For this review, take the finished solid that the model builds, in its own axes (mm). Face numbers are marked on the shaded views. A direction names the side the tool comes from. Coordinates: 2 decimals unless noted, no trailing zeros. Loops run counter-clockwise (first coordinate to the right, second up) from the corner with the lowest first, then second, coordinate; pieces in that order, holes last. Notation, with made-up numbers: M -24,74.5 L -4,74.5 A20 ccw -4,91.5 Z; hole C 24.25,25.25 d8. An arc over 180 degrees is marked long. Answer as a JSON object with one key per item and string values. Group by question number.
Item 1: Wall thickness on L1, parallel to Z at x = 8, y = -19.5; L2, parallel to Y at x = 38, z = 17.5; L3, parallel to X at y = -11, z = 24: over which ranges is each line inside the solid? List them lowest first. Write a range as from..to.
Item 2: Tool access review of the marked faces 4 and 5: name each direction out of +Z, -Z, +X, -X, +Y, -Y from which nothing blocks a thin tool from reaching the whole face with its end or side.
Item 3: Add section A-A (y = -20). State the section outline as (x, z) points.
Item 4: Add section B-B (x = -27.5). State the section outline as (y, z) points, then the cut area to 3 significant figures.
Item 5: Add section C-C (x = 3.5). State the section outline as (y, z) points.
Item 6: Mouldability with a two-part tool opening along X and no side actions: class the marked faces 1, 2 and 3 as +X half, -X half, draft (parallel to the pull), parting line (faces both ways), or undercut.
Item 7: Add section D-D (y = 8.5). State the section outline as (x, z) points, then the cut area to 3 significant figures.
Item 8: Insertion check: pin 1 (3 mm diameter, centred on y = -12.5, z = 30.5, fed in from -X); pin 2 (4 mm diameter, centred on y = -21.5, z = 22.5, fed in from +X); pin 3 (10 mm diameter, centred on x = -1.5, y = -19.5, fed in from -Z). Each pin has a flat end and moves straight along its axis. Give the tip position at first contact, or say it passes through.
from build123d import *

# Parameters (mm, degrees)
F1_DEPTH  = 12.7
F2_DEPTH  = 12.7
F3_R      = 3.8439536327
F4_DEPTH  = 25.401
F5_W      = 29.3294070289
F5_H      = 13.9285232872
F6_DEPTH  = 12.7
F8_DEPTH  = 18.6216022351
F9_R      = 3.0824278946
F10_DEPTH = 59.0766736131


with BuildPart() as f1:
    # F0 (on Front) → F1 (new body, symmetric)
    with BuildSketch(Plane.XZ):
        with BuildLine():
            Line((35.185629891, 37.1372154056), (-28.314370109, 37.1372154056))
            ThreePointArc((-28.314370109, 37.1372154056), (-19.6745097456, 33.5584680661), (-16.0957624062, 24.9186077028))
            ThreePointArc((-16.0957624062, 24.9186077028), (-19.6745097456, 16.2787473395), (-28.314370109, 12.7))
            Line((-28.314370109, 12.7), (35.185629891, 12.7))
            ThreePointArc((35.185629891, 12.7), (22.9670221883, 24.9186077028), (35.185629891, 37.1372154056))
        make_face()
        with BuildLine():
            ThreePointArc((47.4042375938, 24.9186077028), (43.8254902544, 33.5584680661), (35.185629891, 37.1372154056))
            ThreePointArc((35.185629891, 37.1372154056), (22.9670221883, 24.9186077028), (35.185629891, 12.7))
            ThreePointArc((35.185629891, 12.7), (43.8254902544, 16.2787473395), (47.4042375938, 24.9186077028))
        make_face()
    extrude(amount=F1_DEPTH, both=True)

    # F0 (on Front) → F2 (join, symmetric)
    with BuildSketch(Plane.XZ):
        with BuildLine():
            ThreePointArc((-16.0957624062, 24.9186077028), (-19.6745097456, 33.5584680661), (-28.314370109, 37.1372154056))
            ThreePointArc((-28.314370109, 37.1372154056), (-40.5329778117, 24.9186077028), (-28.314370109, 12.7))
            ThreePointArc((-28.314370109, 12.7), (-19.6745097456, 16.2787473395), (-16.0957624062, 24.9186077028))
        make_face()
        with BuildLine():
            Line((35.185629891, 37.1372154056), (-28.314370109, 37.1372154056))
            ThreePointArc((-28.314370109, 37.1372154056), (-19.6745097456, 33.5584680661), (-16.0957624062, 24.9186077028))
            ThreePointArc((-16.0957624062, 24.9186077028), (-19.6745097456, 16.2787473395), (-28.314370109, 12.7))
            Line((-28.314370109, 12.7), (35.185629891, 12.7))
            ThreePointArc((35.185629891, 12.7), (22.9670221883, 24.9186077028), (35.185629891, 37.1372154056))
        make_face()
        with BuildLine():
            ThreePointArc((47.4042375938, 24.9186077028), (43.8254902544, 33.5584680661), (35.185629891, 37.1372154056))
            ThreePointArc((35.185629891, 37.1372154056), (22.9670221883, 24.9186077028), (35.185629891, 12.7))
            ThreePointArc((35.185629891, 12.7), (43.8254902544, 16.2787473395), (47.4042375938, 24.9186077028))
        make_face()
    extrude(amount=F2_DEPTH, both=True)

    # F3 (on face) → F4 (cut, through all)
    with BuildSketch(Plane.XZ.offset(12.7)):
        with Locations((-28.314370109, 24.9186077028)):
            Circle(F3_R)
        with Locations((35.185629891, 24.9186077028)):
            Circle(F3_R)
    extrude(amount=-F4_DEPTH, mode=Mode.SUBTRACT)

    # F5 (on face) → F6 (join)
    with BuildSketch(Plane.XZ.offset(12.7)):
        with Locations((2.9932674952, 25.4808748141)):
            Rectangle(F5_W, F5_H)
    extrude(amount=F6_DEPTH)

    # F7 (on face) → F8 (cut, through all)
    with BuildSketch(Plane(origin=(0, 0, 18.5166131705), x_dir=(1, 0, 0), z_dir=(0, 0, -1))):
        with BuildLine():
            Line((7.2608599439, 21.0908427835), (7.2608599439, 25.4))
            Line((7.2608599439, 25.4), (-1.028164872, 25.4))
            Line((-1.028164872, 25.4), (-1.028164872, 21.0908427835))
            ThreePointArc((-1.028164872, 21.0908427835), (3.116347536, 16.9463303755), (7.2608599439, 21.0908427835))
        make_face()
    extrude(amount=-F8_DEPTH, mode=Mode.SUBTRACT)

    # F9 (on face) → F10 (cut, through all)
    with BuildSketch(Plane(origin=(-11.6714360192, 0, 0), x_dir=(0, -1, 0), z_dir=(-1, 0, 0))):
        with Locations((19.5776261389, 25.3012273461)):
            Circle(F9_R)
    extrude(amount=-F10_DEPTH, mode=Mode.SUBTRACT)


solid = f1.part
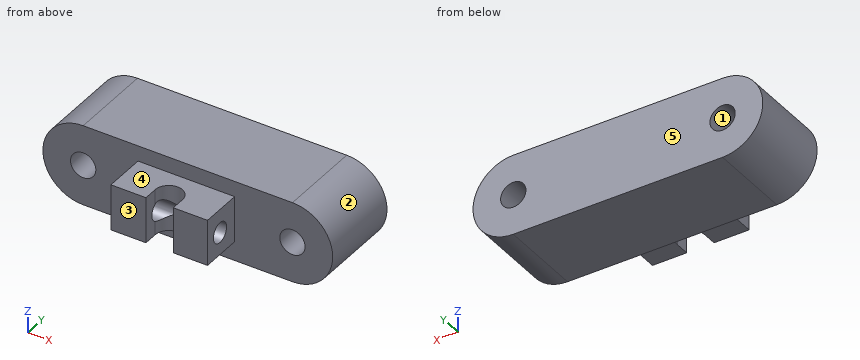
From the geometry:
{
 "1": {"L1": "z = 18.52..22.22, 28.38..32.45", "L2": "y = -12.7..12.7", "L3": "x = -40.5..-32.05, -24.58..31.45, 38.92..47.37"},
 "2": {"face 4": "+Z, +X, -X, -Y", "face 5": "+Z, -Z, +X, -X, +Y"},
 "3": {"outline": "M -11.67,18.52 L -0.88,18.52 L -0.88,22.25 L -11.67,22.25 Z; M -11.67,28.35 L -0.88,28.35 L -0.88,32.45 L -11.67,32.45 Z; M 7.11,18.52 L 17.66,18.52 L 17.66,22.25 L 7.11,22.25 Z; M 7.11,28.35 L 17.66,28.35 L 17.66,32.45 L 7.11,32.45 Z"},
 "4": {"outline": "M -12.7,12.7 L 12.7,12.7 L 12.7,21.16 L -12.7,21.16 Z; M -12.7,28.68 L 12.7,28.68 L 12.7,37.14 L -12.7,37.14 Z", "area": "430 mm²"},
 "5": {"outline": "M -16.96,18.52 L -12.7,18.52 L -12.7,12.7 L 12.7,12.7 L 12.7,37.14 L -12.7,37.14 L -12.7,32.45 L -16.96,32.45 L -16.96,26.94 A3.08 cw -16.96,23.67 Z"},
 "6": {"face 1": "undercut", "face 2": "+X half", "face 3": "draft"},
 "7": {"outline": "M -28.31,12.7 L 35.19,12.7 A12.22 ccw 35.19,37.14 L -28.31,37.14 A12.22 ccw Z; hole C -28.31,24.92 d7.69; hole C 35.19,24.92 d7.69", "area": "1,930 mm²"},
 "8": {"pin 1": "stops at x = -39.83", "pin 2": "stops at x = 17.66", "pin 3": "stops at z = 18.52"}
}
